Can you work these out from the model? Positions are in its coordinate system, mm. Face numbers are marked on the shaded views. A direction names the side the tool comes from. Give positions to 0.01 mm unless a question says otherwise; leave off trailing zeros. Loops run counter-clockwise (first coordinate to the right, second up) from the corner with the lowest first, then second, coordinate; pieces in that order, holes last.
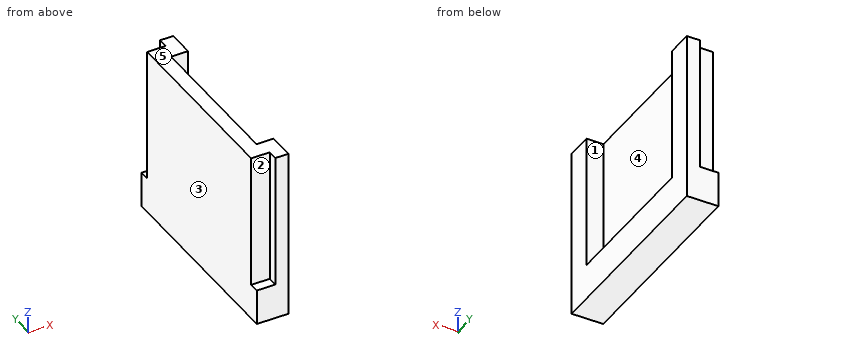
from build123d import *

# Parameters (mm, degrees)
F0_W     = 16.764
F0_H     = 2.5908
F1_DEPTH = 13.97
F2_W     = 0.8128
F2_H     = 1.524
F2_W_2   = 12.446
F2_H_2   = 1.397
F3_DEPTH = 11.049
F4_ANGLE = -90
F5_ANGLE = 90


with BuildPart() as f1:
    # F0 (on Front) → F1 (new body)
    with BuildSketch(Plane.XZ):
        with Locations((8.382, 1.2954)):
            Rectangle(F0_W, F0_H)
    extrude(amount=F1_DEPTH)

    # F2 (on face) → F3 (cut)
    with BuildSketch(Plane(origin=(0, 0, 0), x_dir=(-1, 0, 0), z_dir=(0, 1, 0))):
        with Locations((-16.3576, 1.8288)):
            Rectangle(F2_W, F2_H)
        with Locations((-0.4064, 1.8288)):
            Rectangle(F2_W, F2_H)
        with Locations((-8.382, 0.6985)):
            Rectangle(F2_W_2, F2_H_2)
    extrude(amount=-F3_DEPTH, mode=Mode.SUBTRACT)


with BuildPart() as f1_1:
    # F4: moved
    add(f1.part.rotate(Axis((0, -13.97, 1.2954), (0, 0, 1)), F4_ANGLE))


with BuildPart() as f1_2:
    # F5: moved
    add(f1_1.part.rotate(Axis((0, -22.352, 0), (0, -1, 0)), F5_ANGLE))


solid = f1_2.part
(1) Suppose I cut it at A-A on x = -0.75. List the corners of the cut face in (y, z) for me (3 decimals), plus the area to 3 significant figures.
Returned:
outline: (-30.734, 0) - (-13.97, 0) - (-13.97, 13.97) - (-16.129, 13.97) - (-16.129, 2.921) - (-28.575, 2.921) - (-28.575, 13.97) - (-30.734, 13.97) - close
area: 96.7 mm2
(2) Will these pins go through, and if not, where does the flat tip stop? P1, Ø0.7, axis at x = -1.5, y = -30.5, coming from the +Z side; P2, Ø0.9, axis at x = -2, y = -14.5, coming from the +Z side.
Returned:
P1: stops at z = 2.92
P2: stops at z = 13.97
(3) Please list where these lines run through material, in increasing order: probe 1 along Y at (x, z) = (-0.45, 13) (3 decimals); probe 2 along Y at (x, z) = (-1.3, 4.75) (3 decimals); probe 3 along Z at (x, y) = (-1.1, -17).
Returned:
probe 1: y = -30.734 to -28.575, -16.129 to -13.97
probe 2: y = -29.921 to -28.575, -16.129 to -14.783
probe 3: z = 0 to 2.92
(4) Thinking about a two-plate mould opening in Y: for the marked faces 1, 2 and 3, which applies, pulls with the +Y half, pulls with the -Y half, needs draft (parallel to the pull), parting line crosses it, or undercut?
Returned:
face 1: undercut
face 2: pulls with the -Y half
face 3: needs draft
(5) Suppose I cut it at B-B on y = -18. List the corners of the cut face in (x, z) for me, plus the area to 3 significant figures.
Returned:
outline: (-2.59, 0) - (0, 0) - (0, 2.92) - (-1.4, 2.92) - (-1.4, 13.97) - (-2.59, 13.97) - close
area: 20.8 mm2
(6) Suppose I cut it at D-D on x = -2. List the corners of the cut face in (y, z) for me, plus the area to 3 significant figures.
Returned:
outline: (-30.73, 0) - (-13.97, 0) - (-13.97, 2.92) - (-14.78, 2.92) - (-14.78, 13.97) - (-29.92, 13.97) - (-29.92, 2.92) - (-30.73, 2.92) - close
area: 216 mm2
(7) Which directions (+Z, -Z, +X, -X, +Y, -Y) give clear straight access to the entire face, cutting with the end or side of a thin tool? Please do the marked faces 4 and 5.
Returned:
face 4: +Z, +X
face 5: +Z, +X, -X, +Y, -Y
(8) Suppose I cut it at C-C on z = 7.25. List the corners of the cut face in (x, y) for me (3 decimals), plus the area to 3 significant figures.
Returned:
outline: (-2.591, -29.921) - (-1.067, -29.921) - (-1.067, -30.734) - (0, -30.734) - (0, -28.575) - (-1.397, -28.575) - (-1.397, -16.129) - (0, -16.129) - (0, -13.97) - (-1.067, -13.97) - (-1.067, -14.783) - (-2.591, -14.783) - close
area: 23.6 mm2
